Part model, mm, in its own coordinate system. Face numbers are marked on the shaded views. A direction names the side the tool comes from. Give positions to 0.01 mm unless a question says otherwise; leave off trailing zeros. Write each loop counter-clockwise with the first axis right and the second up, starting at its lowest first coordinate (ties: lowest second). Pieces come first, ordered by that corner, then holes.
Autodesk Inventor part; units mm, degrees
ref_plane "YZ Plane" through (0, 0, 0) normal (1, 0, 0) x (0, 1, 0)
ref_plane "XZ Plane" through (0, 0, 0) normal (0, 1, 0) x (-1, 0, 0)
ref_plane "XY Plane" through (0, 0, 0) normal (0, 0, 1) x (1, 0, 0)
sketch "Skizze1" plane through (0, 0, 0) normal (0, 1, 0) x (-1, 0, 0)
  line L0 (0, 100) -> (0, 100)
  line L1 (-5, 63.8645) -> (-5, 16)
  line L2 (5, 16) -> (5, 63.8645)
  arc A0 (-7.9412, 4.2353) -> (7.9412, 4.2353) centre (0, 0) ccw
  arc A1 (5, 16) -> (7.9412, 4.2353) centre (30, 16) ccw
  arc A2 (-7.9412, 4.2353) -> (-5, 16) centre (-30, 16) ccw
  line L3 (0, -30.8) -> (0, 121.8)
  circle A3 centre (0, 75) radius 2.5
  arc A4 (6.5625, 72.5641) -> (-6.5625, 72.5641) centre (0, 75) ccw
  arc A5 (-5, 63.8645) -> (-6.5625, 72.5641) centre (-30, 63.8645) ccw
  arc A6 (6.5625, 72.5641) -> (5, 63.8645) centre (30, 63.8645) ccw
  point P0 (0, 0)
  point P1 (-5, 7.4833)
  point P2 (5, 7.4833)
  point P3 (-5, 70.101)
  point P4 (5, 70.101)
  dimension "d2" = 18
  dimension "d4" = 25
  dimension "d10" = 0
  dimension "d33" = 5
  dimension "d34" = 5
  dimension "d49" = 75
  dimension "d51" = 5
  dimension "d54" = 14
extrude "Extrusion1" add sketch "Skizze1" along normal blind 10
sketch "Skizze8" plane through (0, 10, 0) normal (0, 1, 0) x (1, 0, 0)
  circle A0 centre (0, 0) radius 6
  dimension "d36" = 12
extrude "Extrusion5" add sketch "Skizze8" along normal blind 5.5
fillet "Rundung3" radius 0.2 1 edges at (-6, 15.5, 0)
fillet "Rundung4" radius 0.2 10 edges at (-5.7464, 10, 9.9366) (-5, 10, 39.9322) (5, 10, 39.9322) (5.7464, 10, 9.9366) (0, 10, -9) (-5.7464, 0, 9.9366) (-5, 0, 39.9322) (5, 0, 39.9322) (5.7464, 0, 9.9366) (0, 0, -9)
sketch "Skizze10" plane through (0, 0, 0) normal (0, -1, 0) x (1, 0, 0)
  circle A0 centre (0, 0) radius 3.65
  dimension "d41" = 7.3
extrude "Extrusion6" cut sketch "Skizze10" against normal blind 3
sketch "Skizze11" plane through (0, 3, 0) normal (0, -1, 0) x (1, 0, 0)
  circle A0 centre (0, 0) radius 1.75
  dimension "d44" = 3.5
extrude "Extrusion7" cut sketch "Skizze11" against normal up to next
fillet "Rundung5" radius 0.2 2 edges at (-1.75, 3, 0) (-3.65, 0, 0)
fillet "Rundung6" radius 0.2 1 edges at (-1.75, 15.5, 0)
extrude "Extrusion8" cut sketch "Skizze1" along normal up to next contours A3 L3 | L3 A3
sketch "Skizze12" plane through (0, 15.5, 0) normal (0, 1, 0) x (1, 0, 0)
  line L0 (0, -83.6989) -> (25.2084, -83.6989)
  line L1 (25.2084, -83.6989) -> (25.2084, 12.8308)
  line L2 (25.2084, 12.8308) -> (0, 12.8308)
  line L3 (0, 12.8308) -> (0, -83.6989)
  point P0 (0, 0)
extrude "Extrusion9" cut sketch "Skizze12" against normal up to next
properties part number "alternativeJoint"
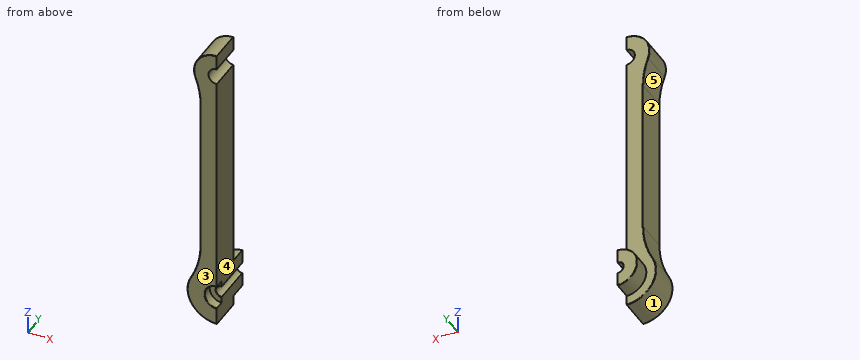
1) 3-axis set-ups, long thin cutter, end or side, ignore diameter. For the marked faces 4 and 5: which of +Z, -Z, +X, -X, +Y, -Y reach the whole face in a straight line?
Answers follow:
face 4: +Z, -Z, +X, +Y, -Y
face 5: -X, +Y, -Y
2) Pin check, flat tips, straight feed: pin 1 Ø2.5 at (x, z) = (-6.5, 48.5) entering from +Y; pin 2 Ø7.5 at (y, z) = (5, 46.5) entering from -X; pin 3 Ø5 at (x, y) = (-6.5, 5.5) entering from +Z. Stop position of each tip, or through.
Answers follow:
pin 1: passes through
pin 2: stops at x = -5
pin 3: stops at z = 80.74
3) Saw through at C-C, the plane z = 44. Write the cut outline in (x, y), then the cut area to 3 significant figures.
Answers follow:
outline: (-5, 0.2) arc R0.2 ccw to (-4.8, 0) - (0, 0) - (0, 10) - (-4.8, 10) arc R0.2 ccw to (-5, 9.8) - close
area: 50.0 mm2
4) Saw through at A-A, the plane y = 4.5. Write the cut outline in (x, z), then the cut area to 3 significant figures.
Answers follow:
outline: (-7.94, 4.24) arc R9 ccw to (0, -9) - (0, -1.75) arc R1.75 cw to (0, 1.75) - (0, 72.5) arc R2.5 cw to (0, 77.5) - (0, 82) arc R7 ccw to (-6.56, 72.56) arc R25 cw to (-5, 63.86) - (-5, 16) arc R25 cw to start
area: 498 mm2
5) Saw through at B-B, the plane z = 0. Write the cut outline in (x, y), then the cut area to 3 significant figures.
Answers follow:
outline: (-9, 0.2) arc R0.2 ccw to (-8.8, 0) - (-3.85, 0) arc R0.2 ccw to (-3.65, 0.2) - (-3.65, 3) - (-1.95, 3) arc R0.2 ccw to (-1.75, 3.2) - (-1.75, 15.3) arc R0.2 ccw to (-1.95, 15.5) - (-5.8, 15.5) arc R0.2 ccw to (-6, 15.3) - (-6, 10) - (-8.8, 10) arc R0.2 ccw to (-9, 9.8) - close
area: 90.1 mm2
6) Wall check: L1, parallel to Z at x = -1.5, y = 5.5; L2, parallel to Z at x = -2, y = 1.25; L3, parallel to Y at x = -0.25, z = 41. Give the ranges that are in metal, low to high.
Answers follow:
L1: z = -8.87 to -0.9, 0.9 to 73, 77 to 81.84
L2: z = -8.77 to -3.05, 3.05 to 73.5, 76.5 to 81.71
L3: y = 0 to 10
7) Saw through at D-D, the plane x = -1. Count the separate pieces of the cut face and the enclosed holes in it, then the cut area to 3 significant figures.
Answers follow:
separate pieces: 3
enclosed holes: 0
area: 871 mm2
8) Two-plate mould, pull along Z, no slides. Class the marked faces 1, 2 and 3: +Z half, -Z half, draft (parallel to the pull), parting line (faces both ways), or undercut.
Answers follow:
face 1: parting line
face 2: undercut
face 3: draft
